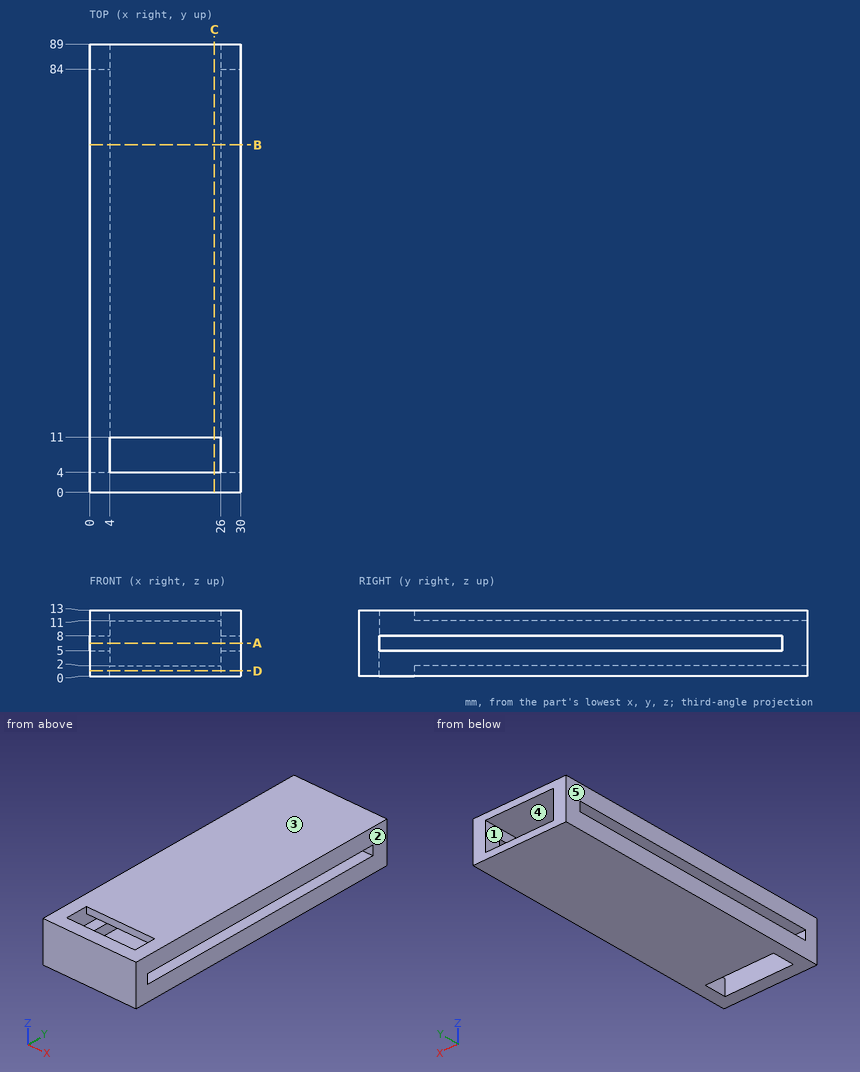
Study the drawing (mm; zero at the part's minimum x, y, z) and answer. A direction names the side the tool comes from. Give positions to 0.01 mm unless a question says otherwise; leave off trailing zeros. Order: outer loops, then holes, each group sorted by start corner. A loop starts at its lowest first (then second) coordinate and runs counter-clockwise, first axis right, second up. Notation, with made-up numbers: (84, -11.75) - (126, -11.75) arc R35 cw to (126, 26.25) - close; hole circle Ø2 at (72.5, -8). An arc over 180 degrees is marked (long way). Answer as CSV lines item,"result". Start each with the question number.
Q1. Given pin 1 Ø1 at (x, z) = (24.5, 3) entering from +Y, flat-ended and moving along its own axis, determine where the tip first touches the part or whether it passes through.
Q2. Find the intervals of material crossed by L1, parallel to Z at x = 28.75, y = 65; L2, parallel to Z at x = 14.25, y = 14; L3, parallel to X at y = 35, z = 8.75, in increasing order. Write a range as [from, to].
Q3. The part is cut by section B-B (y = 69). Write down the section's boundary in (x, z).
Q4. For the marked faces 4 and 5, determine the directions among +Z, -Z, +X, -X, +Y, -Y from which every point of the face is accessible in a straight line to the end or side of a thin tool.
Q5. The part is cut by section C-C (x = 24.75). Write down the section's boundary in (y, z), then the cut area to 3 significant figures.
Q6. The mould has two halves that part along X. Classify the marked faces 1, 2 and 3: +X half, -X half, draft (parallel to the pull), parting line (faces both ways), or undercut.
Q7. The part is cut by section D-D (z = 1). Write down the section's boundary in (x, y), then the cut area to 3 significant figures.
Q8. The part is cut by section A-A (z = 6.5). Write down the section's boundary in (x, y).
Check result:
1,pin 1,"stops at y = 4"
2,L1,"z = [0, 5], [8, 13]"
2,L2,"z = [0, 2], [11, 13]"
2,L3,"x = [0, 4], [26, 30]"
3,outline,"(0, 0) - (30, 0) - (30, 5) - (26, 5) - (26, 2) - (4, 2) - (4, 5) - (0, 5) - close; (0, 8) - (4, 8) - (4, 11) - (26, 11) - (26, 8) - (30, 8) - (30, 13) - (0, 13) - close"
4,face 4,"+Y"
4,face 5,"+Z, -Z, -X, +Y, -Y"
5,outline,"(0, 0) - (4, 0) - (4, 13) - (0, 13) - close; (11, 0) - (89, 0) - (89, 2) - (11, 2) - close; (11, 11) - (89, 11) - (89, 13) - (11, 13) - close"
5,area,"364 mm²"
6,face 1,"undercut"
6,face 2,"+X half"
6,face 3,"draft"
7,outline,"(0, 0) - (30, 0) - (30, 89) - (0, 89) - close; hole (4, 4) - (26, 4) - (26, 11) - (4, 11) - close"
7,area,"2,520 mm²"
8,outline,"(0, 0) - (30, 0) - (30, 4) - (0, 4) - close; (0, 84) - (4, 84) - (4, 89) - (0, 89) - close; (26, 84) - (30, 84) - (30, 89) - (26, 89) - close"
